Read the model definition and answer for the solid it produces. Units are mm, in the model's axes. A direction names the side the tool comes from. Round coordinates to 2 decimals unless told otherwise and drop trailing zeros. Order: outer loops, then holes, each group sorted by start corner. A loop starts at its lowest first (then second) coordinate and runs counter-clockwise, first axis right, second up. Notation, with made-up numbers: (43, 58.25) - (72, 58.25) arc R11 cw to (72, 71.25) - close; hole circle Ø2 at (12.25, -1.5). An arc over 180 degrees is marked (long way). One line per question, with ' | ' between items. Start each with the question number.
1) Flat-ended cylindrical pins translate along their axes: pin 1 (8 mm diameter, centred on y = -0.5, z = 3.5, fed in from +X); pin 2 (1.5 mm diameter, centred on x = 5, z = 16.5, fed in from +Y); pin 3 (1 mm diameter, centred on x = 5, z = 11.5, fed in from -Y); pin 4 (2 mm diameter, centred on x = -4.5, z = 22, fed in from -Y). Find the tip coordinate at first contact, or state that the pin passes through.
2) The part is cut by section A-A, the plane z = 15. Give the vertices of the cut face in (x, y).
3) The part is cut by section C-C, the plane y = 0.5. Give the vertices of the cut face in (x, z), plus the area to 3 significant figures.
4) The part is cut by section B-B, the plane x = -0.25. Give the vertices of the cut face in (y, z).
5) Straight lines are drawn through the part: line 1 (X direction, y = 2.75, z = 21); line 2 (X direction, y = 2.5, z = 25.25); line 3 (X direction, y = -0.5, z = 14.25). For each, find the intervals that lie inside material, in ascending order. Write a range as from..to.
6) The part is cut by section D-D, the plane y = -3. Give the vertices of the cut face in (x, z).
7) The mould has two halves that part along X. Classify faces 6 (the flat face through (12.56, 3, 15)), 7 (the cylindrical face through (12.053, 2.871, 19.995)), 8 (the flat face through (2.835, 1, 15)), 9 (the flat face through (5.835, 7, 15)): pulls with the +X half, pulls with the -X half, needs draft (parallel to the pull), parting line crosses it, or undercut.
8) For faces 1 (the cylindrical face through (10.053, 2.871, 19.995)), 2 (the flat face through (-9, -1.849, 15)), 3 (the flat face through (11.56, 1, 10)), 4 (the flat face through (-7.165, 1, 15)), 5 (the flat face through (-8, 3.151, 15)), determine the directions among +Z, -Z, +X, -X, +Y, -Y from which every point of the face is accessible in a straight line to the end or side of a thin tool.
from build123d import *

# Parameters (mm, degrees)
BOSS_EXTRUDE1_DEPTH = 30
SKETCH3_W           = 10
SKETCH3_H           = 26
CUT_EXTRUDE1_DEPTH  = 5
SKETCH6_R           = 5
BOSS_EXTRUDE2_DEPTH = 1
SKETCH7_R           = 7.5
BOSS_EXTRUDE3_DEPTH = 1
SKETCH8_R           = 5
BOSS_EXTRUDE4_DEPTH = 1


with BuildPart() as part:
    # Sketch1 → Boss-Extrude1 (new body)
    with BuildSketch(Plane.XY):
        Polygon((-14.164814983, 3.151006711), (-14.164814983, -1.848993289), (5.835185017, -1.848993289), (5.835185017, -4.848993289), (9.560017232, -4.848993289), (9.560017232, 10.151006711), (5.835185017, 10.151006711), (5.835185017, 3.151006711), align=None)
    extrude(amount=BOSS_EXTRUDE1_DEPTH)

    # Sketch3 → Cut-Extrude1 (cut)
    with BuildSketch(Plane(origin=(0, 3.151006711, 0), x_dir=(1, 0, 0), z_dir=(0, 1, 0))):
        with Locations((-2.164814983, -15)):
            Rectangle(SKETCH3_W, SKETCH3_H)
    extrude(amount=-CUT_EXTRUDE1_DEPTH, mode=Mode.SUBTRACT)

    # Sketch6 → Boss-Extrude2 (add)
    with BuildSketch(Plane(origin=(9.560017232, 0, 0), x_dir=(0, 0, -1), z_dir=(1, 0, 0))):
        with Locations((-15, 2.651006711)):
            Circle(SKETCH6_R)
    extrude(amount=BOSS_EXTRUDE2_DEPTH)

    # Sketch7 → Boss-Extrude3 (add)
    with BuildSketch(Plane(origin=(10.560017232, 0, 0), x_dir=(0, 0, -1), z_dir=(1, 0, 0))):
        with Locations((-15, 2.651006711)):
            Circle(SKETCH7_R)
    extrude(amount=BOSS_EXTRUDE3_DEPTH)

    # Sketch8 → Boss-Extrude4 (add)
    with BuildSketch(Plane(origin=(11.560017232, 0, 0), x_dir=(0, 0, -1), z_dir=(1, 0, 0))):
        with Locations((-15, 2.651006711)):
            Circle(SKETCH8_R)
    extrude(amount=BOSS_EXTRUDE4_DEPTH)


solid = part.part
Values:
1) pin 1: stops at x = 9.56 | pin 2: stops at y = 3.15 | pin 3: stops at y = -1.85 | pin 4: passes through
2) outline: (-14.16, -1.85) - (-7.16, -1.85) - (-7.16, 3.15) - (-14.16, 3.15) - close; (2.84, -1.85) - (5.84, -1.85) - (5.84, -4.85) - (9.56, -4.85) - (9.56, -2.35) - (10.56, -2.35) - (10.56, -4.85) - (11.56, -4.85) - (11.56, -2.35) - (12.56, -2.35) - (12.56, 7.65) - (11.56, 7.65) - (11.56, 10.15) - (10.56, 10.15) - (10.56, 7.65) - (9.56, 7.65) - (9.56, 10.15) - (5.84, 10.15) - (5.84, 3.15) - (2.84, 3.15) - close
3) outline: (-14.16, 0) - (9.56, 0) - (9.56, 10.49) - (10.56, 10.49) - (10.56, 7.82) - (11.56, 7.82) - (11.56, 10.49) - (12.56, 10.49) - (12.56, 19.51) - (11.56, 19.51) - (11.56, 22.18) - (10.56, 22.18) - (10.56, 19.51) - (9.56, 19.51) - (9.56, 30) - (-14.16, 30) - close; hole (-7.16, 2) - (2.84, 2) - (2.84, 28) - (-7.16, 28) - close | area: 484 mm^2
4) outline: (-1.85, 0) - (3.15, 0) - (3.15, 2) - (-1.85, 2) - close; (-1.85, 28) - (3.15, 28) - (3.15, 30) - (-1.85, 30) - close
5) line 1: x = -14.16..-7.16, 2.84..9.56, 10.56..11.56 | line 2: x = -14.16..-7.16, 2.84..9.56 | line 3: x = -14.16..-7.16, 2.84..12.56
6) outline: (5.84, 0) - (9.56, 0) - (9.56, 30) - (5.84, 30) - close; (10.56, 10.07) - (11.56, 10.07) - (11.56, 19.93) - (10.56, 19.93) - close
7) face 6: pulls with the +X half | face 7: needs draft | face 8: undercut | face 9: pulls with the -X half
8) face 1: none | face 2: +Z, -Z, -X, -Y | face 3: +X | face 4: +Y, -Y | face 5: +Z, -Z, -X, +Y
